from build123d import *

# Parameters (mm, degrees)
SKETCH1_W           = 26.5
SKETCH1_H           = 27.5
BOSS_EXTRUDE1_DEPTH = 12
SKETCH3_W           = 9.5
SKETCH3_H           = 25.5
CUT_EXTRUDE1_DEPTH  = 24.5
SKETCH4_W           = 9
SKETCH4_H           = 9
CUT_EXTRUDE2_DEPTH  = 3.5
SKETCH6_W           = 3
SKETCH6_H           = 27.5
BOSS_EXTRUDE2_DEPTH = 5
SKETCH7_R           = 1
CUT_EXTRUDE3_DEPTH  = 5


with BuildPart() as part:
    # Sketch1 → Boss-Extrude1 (new body)
    with BuildSketch(Plane.XY):
        Rectangle(SKETCH1_W, SKETCH1_H)
    extrude(amount=BOSS_EXTRUDE1_DEPTH)

    # Sketch3 → Cut-Extrude1 (cut)
    with BuildSketch(Plane(origin=(13.25, 0, 0), x_dir=(0, 0, -1), z_dir=(1, 0, 0))):
        with Locations((-6, 0)):
            Rectangle(SKETCH3_W, SKETCH3_H)
    extrude(amount=-CUT_EXTRUDE1_DEPTH, mode=Mode.SUBTRACT)

    # Sketch4 → Cut-Extrude2 (cut)
    with BuildSketch(Plane(origin=(0, 0, 0), x_dir=(-1, 0, 0), z_dir=(0, 0, -1))):
        with Locations((-4.25, 0)):
            Rectangle(SKETCH4_W, SKETCH4_H)
    extrude(amount=-CUT_EXTRUDE2_DEPTH, mode=Mode.SUBTRACT)

    # Sketch6 → Boss-Extrude2 (add)
    with BuildSketch(Plane.XY.offset(12)):
        with Locations((-11.75, 0)):
            Rectangle(SKETCH6_W, SKETCH6_H)
    extrude(amount=BOSS_EXTRUDE2_DEPTH)

    # Sketch7 → Cut-Extrude3 (cut)
    with BuildSketch(Plane(origin=(-10.25, 0, 0), x_dir=(0, 0, -1), z_dir=(1, 0, 0))):
        with Locations(Location((-14.5, -10, 0), (0, 0, 90))):
            Circle(SKETCH7_R)
        with Locations(Location((-14.5, 0, 0), (0, 0, 90))):
            Circle(SKETCH7_R)
        with Locations(Location((-14.5, 10, 0), (0, 0, 90))):
            Circle(SKETCH7_R)
    extrude(amount=-CUT_EXTRUDE3_DEPTH, mode=Mode.SUBTRACT)


solid = part.part
The model under review builds one solid part; all positions refer to its coordinate system, in mm. A direction names the side the tool comes from. Coordinates: 2 decimals unless noted, no trailing zeros. Loops run counter-clockwise (first coordinate to the right, second up) from the corner with the lowest first, then second, coordinate; pieces in that order, holes last. Notation, with made-up numbers: M -31,62.25 L 17,62.25 A10 ccw 17,79.25 Z; hole C -32,56 d6. An arc over 180 degrees is marked long. Put each result on its own line as item: value. Start each with the question number.
Q1. Wall thickness on line 1 (Z direction, x = -10.95, y = 10); line 2 (Z direction, x = 6.5, y = 10); line 3 (X direction, y = 2.25, z = 1): over which ranges is each line inside the solid? List them lowest first.
Q2. Add section C-C (x = 2.5). Write out the cut boundary in (y, z), and give its area (3 significant figures).
Q3. Add section B-B (y = -10). Write out the cut boundary in (x, z), and give its area (4 significant figures).
Q4. Clearance check with flat-ended pins moving along their axes: pin 1 (3 mm diameter, centred on y = 10, z = 14.5, fed in from +X); pin 2 (12 mm diameter, centred on x = -8.5, y = -7, fed in from -Z); pin 3 (1 mm diameter, centred on x = 3.5, y = 7, fed in from +Z); pin 4 (2 mm diameter, centred on x = 7, z = 13.5, fed in from +Y). State where each tip first meets the part, or that it passes through.
Q5. For faces 1 (the flat face through (1, -12.75, 6)), 2 (the flat face through (4, -4.5, 1)), 3 (the flat face through (-10.25, 0, 13)), list the 3-axis set-ups (+Z, -Z, +X, -X, +Y, -Y) from which the entire face can be reached by the end or side of a thin tool; tool diameter is ignored.
Q6. Add section A-A (z = 14.5). Write out the cut boundary in (x, y).
Q7. The part is to be moulded in two halves that separate along Y. For faces 4 (the flat face through (1, 0, 12)), 5 (the flat face through (0, -13.75, 6)), 6 (the flat face through (8.75, 0, 1)), 7 (the flat face through (0, 13.75, 6)), say which applies: +Y half, -Y half, draft (parallel to the pull), parting line (faces both ways), or undercut.
Q8. Add section D-D (x = -2). Write out the cut boundary in (y, z), and give its area (4 significant figures).
Answers:
1. line 1: z = 0 to 1.25, 10.75 to 13.5, 15.5 to 17
1. line 2: z = 0 to 1.25, 10.75 to 12
1. line 3: x = -13.25 to -0.25, 8.75 to 13.25
2. outline: M -13.75,0 L -4.5,0 L -4.5,1.25 L -12.75,1.25 L -12.75,10.75 L 12.75,10.75 L 12.75,1.25 L 4.5,1.25 L 4.5,0 L 13.75,0 L 13.75,12 L -13.75,12 Z
2. area: 76.5 mm^2
3. outline: M -13.25,0 L 13.25,0 L 13.25,1.25 L -11.25,1.25 L -11.25,10.75 L 13.25,10.75 L 13.25,12 L -10.25,12 L -10.25,13.5 L -13.25,13.5 Z; M -13.25,15.5 L -10.25,15.5 L -10.25,17 L -13.25,17 Z
3. area: 94.25 mm^2
4. pin 1: stops at x = -10.25
4. pin 2: stops at z = 0
4. pin 3: stops at z = 12
4. pin 4: passes through
5. face 1: +X
5. face 2: -Z
5. face 3: +Z, +X, +Y, -Y
6. outline: M -13.25,-13.75 L -10.25,-13.75 L -10.25,-11 L -13.25,-11 Z; M -13.25,-9 L -10.25,-9 L -10.25,-1 L -13.25,-1 Z; M -13.25,1 L -10.25,1 L -10.25,9 L -13.25,9 Z; M -13.25,11 L -10.25,11 L -10.25,13.75 L -13.25,13.75 Z
7. face 4: draft
7. face 5: -Y half
7. face 6: undercut
7. face 7: +Y half
8. outline: M -13.75,0 L 13.75,0 L 13.75,12 L -13.75,12 Z; hole M -12.75,1.25 L 12.75,1.25 L 12.75,10.75 L -12.75,10.75 Z
8. area: 87.75 mm^2
